```python
from build123d import *

# Parameters (mm, degrees)
F1_DEPTH = 167.64
F2_R     = 0.429247


with BuildPart() as f1:
    # F0 (on Front) → F1 (new body)
    with BuildSketch(Plane.XZ):
        Polygon((-7.488874, -1.712549), (-5.888674, -1.712549), (-5.888674, 18.099476), (-5.253674, 18.099476), (-5.253674, 19.699676), (-9.456766, 19.699676), (-9.456766, 36.387476), (2.125634, 36.387476), (2.125634, 19.699676), (-2.0828, 19.699676), (-2.0828, 18.099476), (-1.4478, 18.099476), (-1.445737, -1.712549), (0.154463, -1.712382), (0.154463, 18.099476), (3.725834, 18.099476), (3.725834, 37.987676), (-11.056966, 37.987676), (-11.056966, 18.099476), (-7.490937, 18.099476), align=None)
    extrude(amount=F1_DEPTH)

    # F2
    f2_edges = [f1.edges().sort_by_distance(p)[0] for p in [
        (-9.273951, 0, 18.099476),
        (-7.489906, 0, 8.193463),
        (-6.688774, 0, -1.712549),
        (-5.888674, 0, 8.193463),
        (-5.571174, 0, 18.099476),
        (-5.253674, 0, 18.899576),
        (-7.35522, 0, 19.699676),
        (-9.456766, 0, 28.043576),
        (-3.665566, 0, 36.387476),
        (2.125634, 0, 28.043576),
        (0.021417, 0, 19.699676),
        (-2.0828, 0, 18.899576),
        (-1.7653, 0, 18.099476),
        (-1.446769, 0, 8.193463),
        (-0.645637, 0, -1.712466),
        (0.154463, 0, 8.193547),
        (1.940149, 0, 18.099476),
        (3.725834, 0, 28.043576),
        (-3.665566, 0, 37.987676),
        (-11.056966, 0, 28.043576),
        (-9.273951, -167.64, 18.099476),
        (-7.489906, -167.64, 8.193463),
        (-6.688774, -167.64, -1.712549),
        (-5.888674, -167.64, 8.193463),
        (-5.571174, -167.64, 18.099476),
        (-5.253674, -167.64, 18.899576),
        (-7.35522, -167.64, 19.699676),
        (-9.456766, -167.64, 28.043576),
        (-3.665566, -167.64, 36.387476),
        (2.125634, -167.64, 28.043576),
        (0.021417, -167.64, 19.699676),
        (-2.0828, -167.64, 18.899576),
        (-1.7653, -167.64, 18.099476),
        (-1.446769, -167.64, 8.193463),
        (-0.645637, -167.64, -1.712466),
        (0.154463, -167.64, 8.193547),
        (1.940149, -167.64, 18.099476),
        (3.725834, -167.64, 28.043576),
        (-3.665566, -167.64, 37.987676),
        (-11.056966, -167.64, 28.043576),
    ]]
    fillet(f2_edges, radius=F2_R)


solid = f1.part
```
Source: CAD feature listing. Evaluate the final solid. Frame: model axes, mm. A direction names the side the tool comes from. Give positions to 0.01 mm unless a question says otherwise; leave off trailing zeros. Write each loop counter-clockwise with the first axis right and the second up, starting at its lowest first coordinate (ties: lowest second). Pieces come first, ordered by that corner, then holes.
1. Section query A-A (z = 30). Return the cut outline in (x, y), then the cut area to 3 significant figures.
2. Section query B-B (y = -102.5). Return the cut outline in (x, z).
3. First-contact query: pin 1 (8 mm diameter, centred on x = -8, z = 6, fed in from -Y); pin 2 (1.8 mm diameter, centred on x = -10, y = -103.5, fed in from -Z); pin 3 (16 mm diameter, centred on y = -99, z = 8.5, fed in from +X); pin 4 (1.5 mm diameter, centred on x = 0.5, z = 28, fed in from +Y). Flat tips, straight axial feed; report the tip coordinate or a pass-through.
4. Material intervals for line 1 along X through (y, z) = (-153, 0.5); line 2 along Z through (x, y) = (-6.25, -110.5); line 3 along Z through (x, y) = (1.5, -52), sorted ascending.
5. Pull-direction query (Z, two-part tool) for faces 5 (the face through (-4, -83, 37.988)), 6 (the face through (2.126, -83, 28)), 7 (the face through (0.154, -83, 8)); classes: +Z half, -Z half, draft (parallel to the pull), parting line (faces both ways), or undercut.
6. Access query for faces 1 (the face through (-9.457, -83, 28)), 2 (the face through (-9, -83, 18.099)), 3 (the face through (2, -83, 18.099)), 4 (the face through (-5.889, -83, 8)). Directions: +Z, -Z, +X, -X, +Y, -Y. A direction counts if a zero-diameter tool reaches every point of the face in a straight line with its end or side. Return the directions, or none.
Output values:
1. outline: (-11.06, -167.21) arc R0.43 ccw to (-10.63, -167.64) - (-9.89, -167.64) arc R0.43 ccw to (-9.46, -167.21) - (-9.46, -0.43) arc R0.43 ccw to (-9.89, 0) - (-10.63, 0) arc R0.43 ccw to (-11.06, -0.43) - close; (2.13, -167.21) arc R0.43 ccw to (2.55, -167.64) - (3.3, -167.64) arc R0.43 ccw to (3.73, -167.21) - (3.73, -0.43) arc R0.43 ccw to (3.3, 0) - (2.55, 0) arc R0.43 ccw to (2.13, -0.43) - close
1. area: 536 mm2
2. outline: (-11.06, 18.1) - (-7.49, 18.1) - (-7.49, -1.71) - (-5.89, -1.71) - (-5.89, 18.1) - (-5.25, 18.1) - (-5.25, 19.7) - (-9.46, 19.7) - (-9.46, 36.39) - (2.13, 36.39) - (2.13, 19.7) - (-2.08, 19.7) - (-2.08, 18.1) - (-1.45, 18.1) - (-1.45, -1.71) - (0.15, -1.71) - (0.15, 18.1) - (3.73, 18.1) - (3.73, 37.99) - (-11.06, 37.99) - close
3. pin 1: stops at y = -167.64
3. pin 2: stops at z = 18.1
3. pin 3: stops at x = 0.15
3. pin 4: passes through
4. line 1: x = -7.49 to -5.89, -1.45 to 0.15
4. line 2: z = -1.71 to 19.7, 36.39 to 37.99
4. line 3: z = 18.1 to 19.7, 36.39 to 37.99
5. face 5: +Z half
5. face 6: undercut
5. face 7: draft
6. face 1: +Y, -Y
6. face 2: -Z, -X, +Y, -Y
6. face 3: -Z, +X, +Y, -Y
6. face 4: -Z, +Y, -Y
